For this review, take the finished solid that the model builds, in its own axes (mm). Face numbers are marked on the shaded views. A direction names the side the tool comes from. Give positions to 0.01 mm unless a question says otherwise; leave off trailing zeros. Loops run counter-clockwise (first coordinate to the right, second up) from the corner with the lowest first, then second, coordinate; pieces in that order, holes last.
```python
from build123d import *

# Parameters (mm, degrees)
F1_DEPTH = 50.8
F3_D     = 19.05
F2_R     = 3.81
F4_DEPTH = 47.9967516642


with BuildPart() as f1:
    # F0 (on Front) → F1 (new body)
    with BuildSketch(Plane.XZ):
        Polygon((0, 47.9957516642), (0, 0), (50.8, 0), (50.8, 16.0704886385), (111.76, 16.0704886385), (111.76, 29.228876307), (50.8, 29.228876307), (50.8, 47.9957516642), align=None)
    extrude(amount=F1_DEPTH)

    # F3 (through all)
    with Locations(Plane(origin=(0, 0, 0), x_dir=(1, 0, 0), z_dir=(0, 0, -1))):
        with Locations((24.9511450529, 25.4)):
            Hole(F3_D / 2)

    # F2 (on Top) → F4 (cut, through all)
    with BuildSketch(Plane.XY):
        with Locations((63.5, -12.7)):
            Circle(F2_R)
        with Locations((63.5, -38.1)):
            Circle(F2_R)
        with Locations((88.9, -12.7)):
            Circle(F2_R)
        with Locations((88.9, -38.1)):
            Circle(F2_R)
        with BuildLine():
            Line((111.76, -50.8), (111.76, -25.4))
            ThreePointArc((111.76, -25.4), (104.3205122421, -43.3605122421), (86.36, -50.8))
            Line((86.36, -50.8), (88.9, -50.8))
            Line((88.9, -50.8), (111.76, -50.8))
        make_face()
        with BuildLine():
            Line((88.9, 0), (86.36, 0))
            ThreePointArc((86.36, 0), (104.3205122421, -7.4394877579), (111.76, -25.4))
            Line((111.76, -25.4), (111.76, 0))
            Line((111.76, 0), (88.9, 0))
        make_face()
    extrude(amount=F4_DEPTH, mode=Mode.SUBTRACT)


solid = f1.part
```
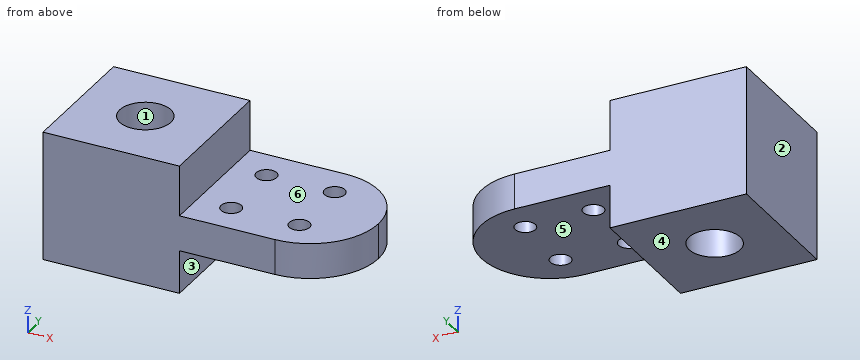
Item 1: Take a section at C-C on y = -29.5. Give the boundary of the cut face in (x, z), and give its area (3 significant figures).
Answer:
outline: (0, 0) - (16.35, 0) - (16.35, 48) - (0, 48) - close; (33.55, 0) - (50.8, 0) - (50.8, 16.07) - (111.43, 16.07) - (111.43, 29.23) - (50.8, 29.23) - (50.8, 48) - (33.55, 48) - close
area: 2,410 mm2
Item 2: Take a section at A-A on x = 63.5. Give the boundary of the cut face in (y, z), and give its area (3 significant figures).
Answer:
outline: (-50.8, 16.07) - (-41.91, 16.07) - (-41.91, 29.23) - (-50.8, 29.23) - close; (-34.29, 16.07) - (-16.51, 16.07) - (-16.51, 29.23) - (-34.29, 29.23) - close; (-8.89, 16.07) - (0, 16.07) - (0, 29.23) - (-8.89, 29.23) - close
area: 468 mm2
Item 3: For L1, parallel to X at y = -35, z = 23; L2, parallel to X at y = -12.7, z = 23.5; L3, parallel to Y at x = 88.9, z = 21.5, list the stretches that pass through material, from the lowest coordinate up.
Answer:
L1: x = 0 to 61.29, 65.71 to 86.69, 91.11 to 109.88
L2: x = 0 to 59.69, 67.31 to 85.09, 92.71 to 108.36
L3: y = -50.67 to -41.91, -34.29 to -16.51, -8.89 to -0.13
Item 4: Take a section at D-D on y = -12.7. Give the boundary of the cut face in (x, z), and give its area (4 significant figures).
Answer:
outline: (0, 0) - (50.8, 0) - (50.8, 16.07) - (59.69, 16.07) - (59.69, 29.23) - (50.8, 29.23) - (50.8, 48) - (0, 48) - close; (67.31, 16.07) - (85.09, 16.07) - (85.09, 29.23) - (67.31, 29.23) - close; (92.71, 16.07) - (108.36, 16.07) - (108.36, 29.23) - (92.71, 29.23) - close
area: 2,995 mm2
Item 5: The part is to be moulded in two halves that separate along X. For the marked faces 1, 2 and 3, say which applies: released by +X, released by -X, zero draft, split by the parting line, or undercut.
Answer:
face 1: undercut
face 2: released by -X
face 3: released by +X
Item 6: Tool access review of the marked faces 4, 5 and 6: name each direction out of +Z, -Z, +X, -X, +Y, -Y from which nothing blocks a thin tool from reaching the whole face with its end or side.
Answer:
face 4: -Z, +X, -X, +Y, -Y
face 5: -Z, +X, +Y, -Y
face 6: +Z, +X, +Y, -Y
Item 7: Clearance check with flat-ended pins moving along their axes: pin 1 Ø6 at (x, z) = (38, 41) entering from +Y; pin 2 Ø13 at (y, z) = (-21, 11) entering from +X; pin 3 Ø20.5 at (y, z) = (-14, 41) entering from +X; pin 4 Ø9 at (x, y) = (63.5, -12.7) entering from -Z. State where each tip first meets the part, or that it passes through.
Answer:
pin 1: stops at y = 0
pin 2: stops at x = 111.76
pin 3: stops at x = 50.8
pin 4: stops at z = 16.07
Item 8: Take a section at B-B on z = 17.5. Give the boundary of the cut face in (x, y) (3 decimals).
Answer:
outline: (0, -50.8) - (86.36, -50.8) arc R25.4 ccw to (86.36, 0) - (0, 0) - close; hole circle Ø19.05 at (24.951, -25.4); hole circle Ø7.62 at (63.5, -38.1); hole circle Ø7.62 at (63.5, -12.7); hole circle Ø7.62 at (88.9, -38.1); hole circle Ø7.62 at (88.9, -12.7)
